The listing builds one solid part. Answer for the finished solid, in the listing's coordinates (mm). A direction names the side the tool comes from. Coordinates: 2 decimals unless noted, no trailing zeros. Order: outer loops, then holes, each group sorted by start corner. A loop starts at its lowest first (then second) coordinate and runs counter-clockwise, first axis right, second up. Notation, with made-up numbers: (39, 40) -> (72, 40) arc R29 ccw to (72, 69) -> close; hole circle Ø10 at (61.25, 6.5). An arc over 180 degrees is marked (long way). One line per question, with ' | ' between items.
from build123d import *

# Parameters (mm, degrees)
F0_W     = 55.88
F0_H     = 43.18
F1_DEPTH = 6.858
F3_R     = 2.921
F4_DEPTH = 3.94335
F5_DEPTH = 4.826
F6_R     = 3.4925
F7_DEPTH = 25.4


with BuildPart() as f1:
    # F0 (on Top) → F1 (new body)
    with BuildSketch(Plane.XY):
        Rectangle(F0_W, F0_H)
    extrude(amount=F1_DEPTH)

    # F3 (on face) → F4 (cut)
    with BuildSketch(Plane(origin=(0, 0, 0), x_dir=(1, 0, 0), z_dir=(0, 0, -1))):
        with Locations((0, 13.97)):
            Circle(F3_R)
    extrude(amount=-F4_DEPTH, mode=Mode.SUBTRACT)

    # F2 (on face) → F5 (cut)
    with BuildSketch(Plane.XY.offset(6.858)):
        Polygon((3.37288, -5.842), (6.745761, 0), (3.37288, 5.842), (-3.37288, 5.842), (-6.745761, 0), (-3.37288, -5.842), align=None)
    extrude(amount=-F5_DEPTH, mode=Mode.SUBTRACT)

    # F6 (on face) → F7 (cut)
    with BuildSketch(Plane.XY.offset(2.032)):
        Circle(F6_R)
    extrude(amount=-F7_DEPTH, mode=Mode.SUBTRACT)


solid = f1.part
Item 1: For faces 5 (the face through (-0.633, -11.118, 1.944)), 6 (the face through (-27.94, 0, 3)), 7 (the face through (5.036, -2.962, 4.479)), determine the directions among +Z, -Z, +X, -X, +Y, -Y from which every point of the face is accessible in a straight line to the end or side of a thin tool.
Computed values:
face 5: -Z | face 6: +Z, -Z, -X, +Y, -Y | face 7: +Z
Item 2: Determine the mould class of faces 1 (the face through (-7, 0, 6.858)), 2 (the face through (-5.036, 2.962, 4.479)), 3 (the face through (0, 21.59, 3)), 4 (the face through (0, -21.59, 3)) for opening direction Y: pulls with the +Y half, pulls with the -Y half, needs draft (parallel to the pull), parting line crosses it, or undercut.
Computed values:
face 1: needs draft | face 2: undercut | face 3: pulls with the +Y half | face 4: pulls with the -Y half
Item 3: Each of these flat-tipped pins is pushed along its axis until it touches: pin 1 Ø4 at (x, y) = (0, 0) entering from -Z; pin 2 Ø1.8 at (x, y) = (0, -15) entering from -Z. Where does it stop, or does it pass through?
Computed values:
pin 1: passes through | pin 2: stops at z = 3.94
Item 4: Section A-A, the plane x = 0 is taken. Give the vertices of the cut face in (y, z), plus the area to 3 significant figures.
Computed values:
outline: (-21.59, 0) -> (-16.89, 0) -> (-16.89, 3.94) -> (-11.05, 3.94) -> (-11.05, 0) -> (-3.49, 0) -> (-3.49, 2.03) -> (-5.84, 2.03) -> (-5.84, 6.86) -> (-21.59, 6.86) -> close; (3.49, 0) -> (21.59, 0) -> (21.59, 6.86) -> (5.84, 6.86) -> (5.84, 2.03) -> (3.49, 2.03) -> close | area: 203 mm^2
Item 5: Section C-C, the plane z = 5.5 is taken. Give the vertices of the cut face in (x, y).
Computed values:
outline: (-27.94, -21.59) -> (27.94, -21.59) -> (27.94, 21.59) -> (-27.94, 21.59) -> close; hole (-6.75, 0) -> (-3.37, -5.84) -> (3.37, -5.84) -> (6.75, 0) -> (3.37, 5.84) -> (-3.37, 5.84) -> close
Item 6: Section B-B, the plane y = -13.97 is taken. Give the vertices of the cut face in (x, z), plus the area to 3 significant figures.
Computed values:
outline: (-27.94, 0) -> (-2.92, 0) -> (-2.92, 3.94) -> (2.92, 3.94) -> (2.92, 0) -> (27.94, 0) -> (27.94, 6.86) -> (-27.94, 6.86) -> close | area: 360 mm^2
Item 7: Find the intervals of material crossed by L1, parallel to Y at x = 0, z = 1; L2, parallel to Y at x = 0, z = 2.4; L3, parallel to X at y = -13.97, z = 2.9, in increasing order.
Computed values:
L1: y = -21.59 to -16.89, -11.05 to -3.49, 3.49 to 21.59 | L2: y = -21.59 to -16.89, -11.05 to -5.84, 5.84 to 21.59 | L3: x = -27.94 to -2.92, 2.92 to 27.94
